Could you check a few things on this model? Use its own coordinates, in mm. A direction names the side the tool comes from. Give positions to 0.01 mm unless a question says otherwise; leave off trailing zeros. Loops run counter-clockwise (first coordinate to the right, second up) from the corner with the lowest first, then second, coordinate; pieces in that order, holes last. Notation, with made-up numbers: (47.25, 34.25) - (80.25, 34.25) arc R10 ccw to (80.25, 38.25) - close; hole circle Ø7 at (8, 42.5). An arc over 180 degrees is marked (long way). Write each question's results on one line, items separated by ' | '. Start each with the question number.
1) If I drill on probe 1 along Z at (x, y) = (1.5, -1.25); probe 2 along Z at (x, y) = (-2.5, 2.5); probe 3 along Y at (x, z) = (0, 25), over which ranges is the centre line in solid material (lowest first)? Write a range as [from, to].
2) I want a section at A-A, the plane x = 0. Write out the boundary of the cut face in (y, z), and give its area (3 significant figures).
3) I'm going to push flat-ended pins straight in: pin 1 (1 mm diameter, centred on x = 3.5, z = 27, fed in from -Y); pin 2 (2 mm diameter, centred on x = -4.5, y = 1, fed in from -Z); pin 3 (1 mm diameter, centred on y = 2.5, z = 9.5, fed in from +X); pin 4 (2.5 mm diameter, centred on x = 0.5, z = 27.5, fed in from +Y). Where does each tip first touch, or does it pass through?
4) I want a section at D-D, the plane x = -4. Write out the boundary of the cut face in (y, z).
5) I want a section at C-C, the plane z = 16. Write out the boundary of the cut face in (x, y), and give its area (3 significant figures).
6) On a 3-axis mill with a long thin cutter (end or side, diameter ignored), from which of +Z, -Z, +X, -X, +Y, -Y can I reach the whole of each face in a straight line? I mean faces 4 (the face through (0.54, 2.44, -1.25)), 5 (the face through (-6, 0, 7)), 6 (the face through (-4.4, 2.7, 16)). Say none if no direction works.
7) If we mould it in two halves opening along Z, with no side actions, what happens to faces 1 (the face through (5.95, -0.08, -0.49)), 2 (the face through (3.935, -3.496, 15.986)), 3 (the face through (-5, 4, 14))? For each: +Z half, -Z half, draft (parallel to the pull), parting line (faces both ways), or undercut.
8) I want a section at B-B, the plane y = 4. Write out the boundary of the cut face in (x, z).
Autodesk Inventor part; units mm, degrees
ref_plane "YZ Plane" through (0, 0, 0) normal (1, 0, 0) x (0, 1, 0)
ref_plane "XZ Plane" through (0, 0, 0) normal (0, 1, 0) x (-1, 0, 0)
ref_plane "XY Plane" through (0, 0, 0) normal (0, 0, 1) x (1, 0, 0)
sketch "Sketch1" plane through (0, 0, 0) normal (0, 0, 1) x (1, 0, 0)
  circle A0 centre (0, 0) radius 6
  line L0 (0, 0) -> (0, 5)
  line L1 (0, 5) -> (3.3166, 5)
  line L2 (0, 5) -> (-3.3166, 5)
  line L3 (0, 0) -> (0, -5)
  line L4 (0, -5) -> (3.3166, -5)
  line L5 (0, -5) -> (-3.3166, -5)
  dimension "d0" = 12
  dimension "d1" = 5
  dimension "d2" = 5
extrude "Extrusion1" add sketch "Sketch1" along normal blind 14 contours A0 L4 L3 L0 L1 | L2 L0 L3 L5 A0
sketch "Sketch2" plane through (0, 0, 14) normal (0, 0, 1) x (1, 0, 0)
  arc A0 (-3.3166, 5) -> (-3.3166, -5) centre (0, 0) ccw
  line L0 (-6, 0) -> (-6, 4.5)
  line L1 (-5.5, 5) -> (5.5, 5)
  line L2 (6, 4.5) -> (6, -4.5)
  line L3 (5.5, -5) -> (-5.5, -5)
  line L4 (-6, -4.5) -> (-6, 5)
  arc A1 (-5.5, 5) -> (-6, 4.5) centre (-5.5, 4.5) ccw
  arc A2 (-6, -4.5) -> (-5.5, -5) centre (-5.5, -4.5) ccw
  arc A3 (5.5, -5) -> (6, -4.5) centre (5.5, -4.5) ccw
  arc A4 (6, 4.5) -> (5.5, 5) centre (5.5, 4.5) ccw
  point P0 (6, -5)
  point P1 (-6, -5)
  dimension "d5" = 12
  dimension "d6" = 0.5
  dimension "d32" = 10
  dimension "d33" = 5
extrude "Extrusion2" add sketch "Sketch2" along normal blind 1
sketch "Sketch3" plane through (0, 0, 15) normal (0, 0, 1) x (1, 0, 0)
  line L0 (0, 0) -> (-4, 0)
  line L1 (-4, 0) -> (-4, 3)
  line L2 (0, 0) -> (0, -3)
  line L3 (0, -3) -> (4, -3)
  circle A0 centre (-4, 3) radius 0.5
  circle A1 centre (4, -3) radius 0.5
  dimension "d9" = 4
  dimension "d10" = 3
  dimension "d11" = 3
  dimension "d12" = 4
  dimension "d13" = 1
  dimension "d14" = 1
extrude "Extrusion3" add sketch "Sketch3" along normal blind 2
sketch "Sketch4" plane through (-4, 3, 17) normal (0, 0, 1) x (1, 0, 0)
  line L0 (-1.5, 2) -> (9.5, 2)
  line L1 (10, 1.5) -> (10, -7.5)
  line L2 (9.5, -8) -> (-1.5, -8)
  line L3 (-2, -7.5) -> (-2, 1.5)
  arc A0 (-1.5, 2) -> (-2, 1.5) centre (-1.5, 1.5) ccw
  arc A1 (-2, -7.5) -> (-1.5, -8) centre (-1.5, -7.5) ccw
  arc A2 (9.5, -8) -> (10, -7.5) centre (9.5, -7.5) ccw
  arc A3 (10, 1.5) -> (9.5, 2) centre (9.5, 1.5) ccw
  line L4 (-1.5, -8) -> (9.5, -8)
  line L5 (-2, 1.5) -> (-2, -7.5)
  point P0 (4, -3)
  dimension "d17" = 0.5
  dimension "d36" = 10
  dimension "d37" = 12
  dimension "d38" = 0
  dimension "d39" = 0
extrude "Extrusion4" add sketch "Sketch4" along normal blind 1
sketch "Sketch5" plane through (-4, 3, 18) normal (0, 0, 1) x (1, 0, 0)
  circle A0 centre (0, 0) radius 0.5
  circle A1 centre (0, 0) radius 0.5
  circle A2 centre (8, -6) radius 0.5
  circle A3 centre (8, -6) radius 0.5
  point P0 (4, -3)
  point P1 (7.9, -5.5101)
  point P2 (7.9, -6.4899)
extrude "Extrusion5" add sketch "Sketch5" along normal blind 4
sketch "Sketch6" plane through (-4, 3, 22) normal (0, 0, 1) x (1, 0, 0)
  line L0 (-1.5, 2) -> (9.5, 2)
  line L1 (10, 1.5) -> (10, -7.5)
  line L2 (9.5, -8) -> (-1.5, -8)
  line L3 (-2, -7.5) -> (-2, 1.5)
  arc A0 (-1.5, 2) -> (-2, 1.5) centre (-1.5, 1.5) ccw
  arc A1 (10, 1.5) -> (9.5, 2) centre (9.5, 1.5) ccw
  arc A2 (9.5, -8) -> (10, -7.5) centre (9.5, -7.5) ccw
  arc A3 (-2, -7.5) -> (-1.5, -8) centre (-1.5, -7.5) ccw
  line L4 (-1.5, -8) -> (9.5, -8)
  line L5 (-2, 1.5) -> (-2, -7.5)
  point P0 (4, -3)
  dimension "d22" = 0.5
  dimension "d40" = 10
  dimension "d41" = 12
  dimension "d42" = 0
  dimension "d43" = 0
extrude "Extrusion6" add sketch "Sketch6" along normal blind 1
sketch "Sketch7" plane through (-4, 3, 23) normal (0, 0, 1) x (1, 0, 0)
  circle A0 centre (4, -3) radius 1.5
  line L0 (4, -3) -> (4, -2)
  line L1 (4, -2) -> (5.118, -2)
  line L2 (4, -2) -> (2.882, -2)
  dimension "d25" = 3
  dimension "d26" = 1
extrude "Extrusion7" add sketch "Sketch7" along normal blind 10 contours A0 L2 L1 picked at (3.9981, -3.6594)
sketch "Sketch8" plane through (0, 0, 0) normal (0, 0, -1) x (-1, 0, 0)
  circle A0 centre (0, 0) radius 5.95
  line L0 (0, 0) -> (0, -5)
  line L1 (3.3166, -5) -> (-3.3166, -5)
  line L2 (0, -5) -> (3.3166, -5)
  line L3 (3.3166, -5) -> (-3.2253, -5)
  line L4 (0, 0) -> (0, 5)
  line L5 (-3.3166, 5) -> (3.3166, 5)
  line L6 (3.289, 4.9583) -> (-3.289, 4.9583)
  point P0 (-3.2253, -5)
  point P1 (3.2253, -5)
  point P2 (3.2253, 5)
  point P3 (-3.2253, 5)
  dimension "d35" = 11.9
  dimension "d34" = 5
extrude "Extrusion8" add sketch "Sketch8" along normal blind 1 contours A0 L1 L0 L4 L6 | L6 L4 L5 A0 | L6 A0 L5 L4 | L4 L0 L1 A0 L6
sketch "Sketch9" plane through (0, 0, -1) normal (0, 0, -1) x (-1, 0, 0)
  arc A0 (-1.118, 1) -> (1.118, 1) centre (0, 0) ccw
  circle A1 centre (0, 0) radius 2.5
  dimension "d44" = 5
extrude "Extrusion9" add sketch "Sketch9" along normal blind 0.5
sketch "Sketch10" plane through (0, 0, -1.5) normal (0, 0, -1) x (-1, 0, 0)
  circle A0 centre (0, 0) radius 0.5
  dimension "d47" = 1
extrude "Extrusion10" add sketch "Sketch10" along normal blind 0.5
properties part number "minimotor"
Answers:
1) probe 1: z = [-1.5, 15], [17, 18], [22, 23] | probe 2: z = [-1, 15], [17, 18], [22, 23] | probe 3: y = [-1.5, 1]
2) outline: (-5, -1) - (-2.5, -1) - (-2.5, -1.5) - (-0.5, -1.5) - (-0.5, -2) - (0.5, -2) - (0.5, -1.5) - (2.5, -1.5) - (2.5, -1) - (5, -1) - (5, 15) - (-5, 15) - close; (-5, 17) - (5, 17) - (5, 18) - (-5, 18) - close; (-5, 22) - (5, 22) - (5, 23) - (1, 23) - (1, 33) - (-1.5, 33) - (-1.5, 23) - (-5, 23) - close | area: 208 mm2
3) pin 1: passes through | pin 2: stops at z = -1 | pin 3: stops at x = 5.66 | pin 4: stops at y = 1
4) outline: (-5, 14) - (-4.47, 14) - (-4.47, 0) - (-4.4, 0) - (-4.4, -1) - (4.4, -1) - (4.4, 0) - (4.47, 0) - (4.47, 14) - (5, 14) - (5, 15) - (3.5, 15) - (3.5, 17) - (5, 17) - (5, 18) - (3.5, 18) - (3.5, 22) - (5, 22) - (5, 23) - (-5, 23) - (-5, 22) - (2.5, 22) - (2.5, 18) - (-5, 18) - (-5, 17) - (2.5, 17) - (2.5, 15) - (-5, 15) - close
5) outline: circle Ø1 at (-4, 3); circle Ø1 at (4, -3) | area: 1.57 mm2
6) face 4: -Z | face 5: -Z, -X | face 6: none
7) face 1: draft | face 2: undercut | face 3: -Z half
8) outline: (-6, 14) - (-4.47, 14) - (-4.47, 0) - (-4.4, 0) - (-4.4, -1) - (4.4, -1) - (4.4, 0) - (4.47, 0) - (4.47, 14) - (6, 14) - (6, 15) - (-6, 15) - close; (-6, 17) - (6, 17) - (6, 18) - (-6, 18) - close; (-6, 22) - (6, 22) - (6, 23) - (-6, 23) - close
